Autodesk Inventor part; units mm, degrees
ref_plane "YZ Plane" through (0, 0, 0) normal (1, 0, 0) x (0, 1, 0)
ref_plane "XZ Plane" through (0, 0, 0) normal (0, 1, 0) x (-1, 0, 0)
ref_plane "XY Plane" through (0, 0, 0) normal (0, 0, 1) x (1, 0, 0)
sketch "スケッチ1" plane through (0, 0, 0) normal (0, 0, 1) x (1, 0, 0)
  line L0 (-13.6656, 4.2556) -> (32.3344, 4.2556)
  line L1 (32.3344, 4.2556) -> (32.3344, -4.7444)
  line L2 (32.3344, -4.7444) -> (-13.6656, -4.7444)
  line L3 (-13.6656, -4.7444) -> (-13.6656, 4.2556)
  point P0 (0, 0)
  dimension "d0" = 46
  dimension "d1" = 9
extrude "押し出し1" add sketch "スケッチ1" along normal blind 3
sketch "スケッチ2" plane through (0, 0, 3) normal (0, 0, 1) x (1, 0, 0)
  line L0 (-10.1656, -0.2444) -> (4.8344, -0.2444) construction
  line L1 (-10.1656, -1.7444) -> (4.8344, -1.7444)
  line L2 (4.8344, 1.2556) -> (-10.1656, 1.2556)
  arc A0 (-10.1656, 1.2556) -> (-10.1656, -1.7444) centre (-10.1656, -0.2444) ccw
  arc A1 (4.8344, -1.7444) -> (4.8344, 1.2556) centre (4.8344, -0.2444) ccw
  line L3 (-13.6656, 4.2556) -> (-13.6656, -4.7444)
  line L4 (32.3344, 4.2556) -> (-13.6656, 4.2556)
  point P0 (0, 0)
  point P1 (-2.6656, -0.2444)
  dimension "d4" = 15
  dimension "d5" = 3
  dimension "d6" = 3.5
  dimension "d7" = 4.5
extrude "押し出し2" cut sketch "スケッチ2" against normal blind 3
equation "\"BendRadius\" = Thickness"
equation "\"BendReliefWidth\" = Thickness"
equation "\"BendReliefDepth\" = 0.5 * Thickness"
equation "\"CornerReliefSize\" = 4 * Thickness"
equation "\"MinimumRemnant\" = 2 * Thickness"
equation "\"TransitionRadius\" = BendRadius"
equation "\"JacobiRadiusSize\" = BendRadius"
equation "\"GapSize\" = Thickness"
properties part number "creat2"
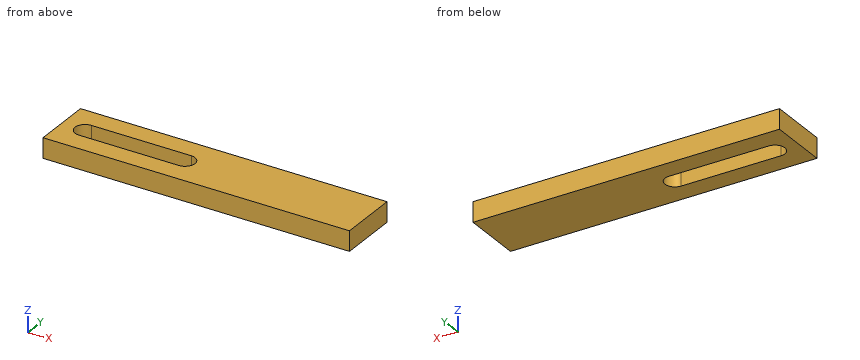
Design review of the part built by this model. Coordinates are the model's own, in mm. Give positions to 0.01 mm unless a question says otherwise; leave off trailing zeros. Write each loop counter-clockwise with the first axis right and the second up, starting at its lowest first coordinate (ties: lowest second). Pieces come first, ordered by that corner, then holes. Notation, with made-up numbers: M 75.25,81.5 L 109.25,81.5 A20 cw 109.25,87.5 Z; hole C 68,7 d4. An arc over 180 degrees is marked long. Return JSON: item names as keys, results as strings. Group by question number.
Item 1: Wall thickness on line 1 along Y through (x, z) = (2.5, 2.65); line 2 along X through (y, z) = (0, 2.1); line 3 along X through (y, z) = (1, 0.55): over which ranges is each line inside the solid? List them lowest first.
Item 2: Clearance check with a flat-ended pin moving along its axis: pin 1 Ø4 at (x, y) = (-7.5, -1) entering from -Z. State where the tip first meets the part, or that it passes through.
Item 3: Take a section at A-A (z = 2.4). Give the boundary of the cut face in (x, y).
Item 4: Take a section at B-B (y = 0). Give the boundary of the cut face in (x, z).
Return value:
{
 "1": {"line 1": "y = -4.74 to -1.74, 1.26 to 4.26", "line 2": "x = -13.67 to -11.65, 6.31 to 32.33", "line 3": "x = -13.67 to -11, 5.67 to 32.33"},
 "2": {"pin 1": "stops at z = 0"},
 "3": {"outline": "M -13.67,-4.74 L 32.33,-4.74 L 32.33,4.26 L -13.67,4.26 Z; hole M -10.17,-1.74 L 4.83,-1.74 A1.5 ccw 4.83,1.26 L -10.17,1.26 A1.5 ccw Z"},
 "4": {"outline": "M -13.67,0 L -11.65,0 L -11.65,3 L -13.67,3 Z; M 6.31,0 L 32.33,0 L 32.33,3 L 6.31,3 Z"}
}
